Build history of the part. All positions in model axes, mm. Coordinates: 2 decimals unless noted, no trailing zeros. Loops run counter-clockwise (first coordinate to the right, second up) from the corner with the lowest first, then second, coordinate; pieces in that order, holes last.
(1) Wall check: L1, parallel to Y at x = 7, z = 31; L2, parallel to X at y = -7.25, z = 62; L3, parallel to X at y = 3, z = 50.5. Give the ranges that are in metal, low to high.
(2) Slice it at A-A (y = 7). Give the cut face in (x, z).
(3) Slice it at B-B (x = 0). Give the cut face in (y, z), and give its area (3 significant figures).
from build123d import *

# Parameters (mm, degrees)
SKETCH_1_W          = 20
SKETCH_1_H          = 20
EXTRUDE_1_DEPTH     = 74.5
SKETCH_2_R          = 2.15
SKETCH_2_R_2        = 2
CUT_EXTRUDE_1_DEPTH = 315.5


with BuildPart() as part:
    # 스케치1 → 보스-돌출1 (new body)
    with BuildSketch(Plane.XY):
        Rectangle(SKETCH_1_W, SKETCH_1_H)
    extrude(amount=EXTRUDE_1_DEPTH)

    # 스케치2 → 컷-돌출1 (cut)
    with BuildSketch(Plane.XY.offset(74.5)):
        Circle(SKETCH_2_R)
        with Locations((-7, 7)):
            Circle(SKETCH_2_R_2)
        with Locations((7, 7)):
            Circle(SKETCH_2_R_2)
        with Locations((7, -7)):
            Circle(SKETCH_2_R_2)
        with Locations((-7, -7)):
            Circle(SKETCH_2_R_2)
        with BuildLine():
            Line((-2.65, 10), (-2.65, 8.5))
            Line((-2.65, 8.5), (-4.15, 8.5))
            Line((-4.15, 8.5), (-4.15, 5.5))
            ThreePointArc((-4.15, 5.5), (0, 4.339407869), (4.15, 5.5))
            Line((4.15, 5.5), (4.15, 8.5))
            Line((4.15, 8.5), (2.65, 8.5))
            Line((2.65, 8.5), (2.65, 10))
            Line((2.65, 10), (-2.65, 10))
        make_face()
        with BuildLine():
            Line((10, 2.65), (8.5, 2.65))
            Line((8.5, 2.65), (8.5, 4.15))
            Line((8.5, 4.15), (5.5, 4.15))
            ThreePointArc((5.5, 4.15), (4.339407869, 0), (5.5, -4.15))
            Line((5.5, -4.15), (8.5, -4.15))
            Line((8.5, -4.15), (8.5, -2.65))
            Line((8.5, -2.65), (10, -2.65))
            Line((10, -2.65), (10, 2.65))
        make_face()
        with BuildLine():
            Line((2.65, -10), (2.65, -8.5))
            Line((2.65, -8.5), (4.15, -8.5))
            Line((4.15, -8.5), (4.15, -5.5))
            ThreePointArc((4.15, -5.5), (0, -4.339407869), (-4.15, -5.5))
            Line((-4.15, -5.5), (-4.15, -8.5))
            Line((-4.15, -8.5), (-2.65, -8.5))
            Line((-2.65, -8.5), (-2.65, -10))
            Line((-2.65, -10), (2.65, -10))
        make_face()
        with BuildLine():
            Line((-10, -2.65), (-8.5, -2.65))
            Line((-8.5, -2.65), (-8.5, -4.15))
            Line((-8.5, -4.15), (-5.5, -4.15))
            ThreePointArc((-5.5, -4.15), (-4.339407869, 0), (-5.5, 4.15))
            Line((-5.5, 4.15), (-8.5, 4.15))
            Line((-8.5, 4.15), (-8.5, 2.65))
            Line((-8.5, 2.65), (-10, 2.65))
            Line((-10, 2.65), (-10, -2.65))
        make_face()
    extrude(amount=-CUT_EXTRUDE_1_DEPTH, mode=Mode.SUBTRACT)


solid = part.part
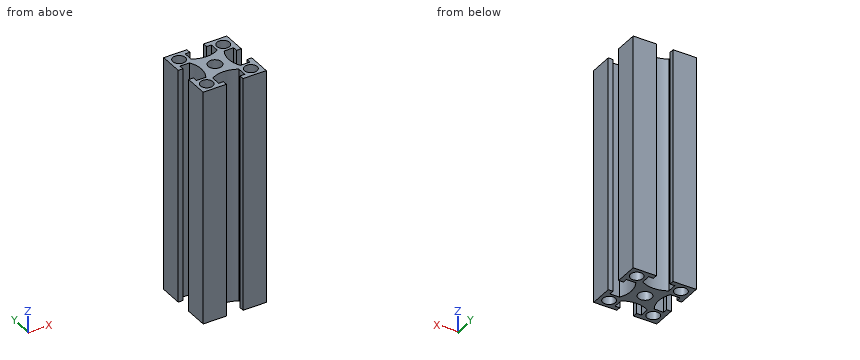
Response values:
1. L1: y = -10 to -9, -5 to -4.15, 4.15 to 5, 9 to 10
1. L2: x = -10 to -8.98, -5.02 to -4.15, 4.15 to 5.02, 8.98 to 10
1. L3: x = -10 to -8.5, -4.92 to 4.92, 8.5 to 10
2. outline: (-10, 0) - (-9, 0) - (-9, 74.5) - (-10, 74.5) - close; (-5, 0) - (-4.15, 0) - (-4.15, 74.5) - (-5, 74.5) - close; (4.15, 0) - (5, 0) - (5, 74.5) - (4.15, 74.5) - close; (9, 0) - (10, 0) - (10, 74.5) - (9, 74.5) - close
3. outline: (-4.34, 0) - (-2.15, 0) - (-2.15, 74.5) - (-4.34, 74.5) - close; (2.15, 0) - (4.34, 0) - (4.34, 74.5) - (2.15, 74.5) - close
3. area: 326 mm2
